```python
from build123d import *

# Parameters (mm, degrees)
SKETCH1_R           = 98.5
SKETCH1_R_2         = 96
BOSS_EXTRUDE1_DEPTH = 38
SKETCH2_W           = 20
SKETCH2_H           = 11
CUT_EXTRUDE1_DEPTH  = 99.5
CIRPATTERN1_COUNT   = 13


with BuildPart() as part:
    # Sketch1 → Boss-Extrude1 (new body)
    with BuildSketch(Plane(origin=(0, 0, 0), x_dir=(1, 0, 0), z_dir=(0, 1, 0))):
        Circle(SKETCH1_R)
        Circle(SKETCH1_R_2, mode=Mode.SUBTRACT)
    extrude(amount=BOSS_EXTRUDE1_DEPTH)

    # Sketch2 → Cut-Extrude1 (cut, symmetric)
    with BuildSketch(Plane.XY):
        with Locations((0, 19.5)):
            Rectangle(SKETCH2_W, SKETCH2_H)
    cut_extrude1 = extrude(amount=CUT_EXTRUDE1_DEPTH, both=True, mode=Mode.SUBTRACT)

    # CirPattern1: Cut-Extrude1 ×13 about axis
    cirpattern1_axis = Axis((0, 0, 0), (0, 1, 0))
    for i in range(1, CIRPATTERN1_COUNT):
        add(cut_extrude1.rotate(cirpattern1_axis, i * 360 / CIRPATTERN1_COUNT), mode=Mode.SUBTRACT)


solid = part.part
```
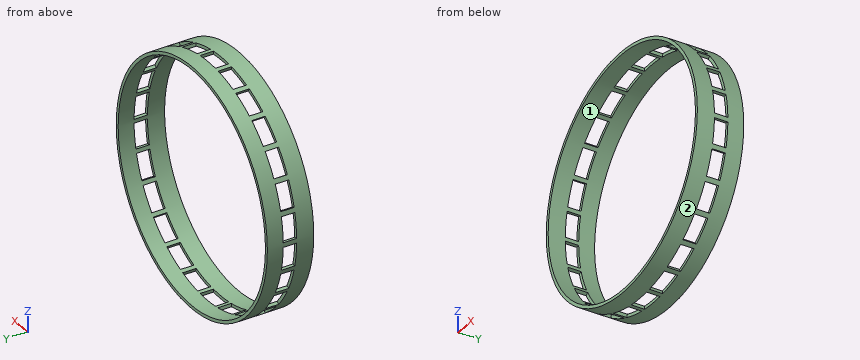
Can you work these out from the model? Positions are in its coordinate system, mm. Face numbers are marked on the shaded views. Round coordinates to 2 decimals unless told otherwise and drop trailing zeros. Loops run counter-clockwise (first coordinate to the right, second up) from the corner with the lowest first, then second, coordinate; pieces in that order, holes last. Notation, with made-up numbers: (-13, -6.75) -> (18, -6.75) arc R17 cw to (18, 19.25) -> close; hole circle Ø8 at (-11.5, 35.5). An arc over 180 degrees is marked (long way). Answer in a Markdown table with one row per item.
Item 1: Will these pins go through, and if not, where does the flat tip stop? P1, Ø8, axis at x = 41.5, y = 5, coming from the +Z side; P2, Ø6, axis at x = -55.5, y = 18.5, coming from the +Z side; P3, Ø12, axis at x = 66.5, y = 26.5, coming from the +Z side.
Answer block:
| item | result |
|---|---|
| P1 | z = 91.08 |
| P2 | z = 82.12 |
| P3 | z = 77.73 |
Item 2: We'd pull the mould along Z, two halves only. Please class the marked faces 1 and 2: released by +Z, released by -Z, zero draft, split by the parting line, or undercut.
Answer block:
| item | result |
|---|---|
| face 1 | undercut |
| face 2 | split by the parting line |
Item 3: If I drill on probe 1 along Z at (x, y) = (-13.5, 10); probe 2 along X at (y, z) = (15, 0), over which ranges is the centre line in solid material (lowest first)?
Answer block:
| item | result |
|---|---|
| probe 1 | -97.57 to -95.05, 95.05 to 97.57 |
| probe 2 | -98.5 to -96, 96 to 98.5 |
Item 4: Suppose I cut it at B-B, the plane z = -58. List the corners of the cut face in (x, y) for me, plus the area to 3 significant figures.
Answer block:
| item | result |
|---|---|
| outline | (-79.61, 0) -> (-76.5, 0) -> (-76.5, 14) -> (-79.61, 14) -> close; (-79.61, 25) -> (-76.5, 25) -> (-76.5, 38) -> (-79.61, 38) -> close; (76.5, 0) -> (79.61, 0) -> (79.61, 14) -> (76.5, 14) -> close; (76.5, 25) -> (79.61, 25) -> (79.61, 38) -> (76.5, 38) -> close |
| area | 168 mm² |
Item 5: Suppose I cut it at A-A, the plane x = 0. List the corners of the cut face in (y, z) for me.
Answer block:
| item | result |
|---|---|
| outline | (0, -98.5) -> (14, -98.5) -> (14, -96) -> (0, -96) -> close; (0, 96) -> (14, 96) -> (14, 98.5) -> (0, 98.5) -> close; (25, -98.5) -> (38, -98.5) -> (38, -96) -> (25, -96) -> close; (25, 96) -> (38, 96) -> (38, 98.5) -> (25, 98.5) -> close |
Item 6: Suppose I cut it at C-C, the plane y = 18. Give the number of separate pieces and of enclosed holes in the cut face, plus the area to 3 significant figures.
Answer block:
| item | result |
|---|---|
| separate pieces | 26 |
| enclosed holes | 0 |
| area | 225 mm² |
Item 7: Suppose I cut it at D-D, the plane y = 4.5. List the corners of the cut face in (x, z) for me.
Answer block:
| item | result |
|---|---|
| outline | circle Ø197 at (0, 0); hole circle Ø192 at (0, 0) |
